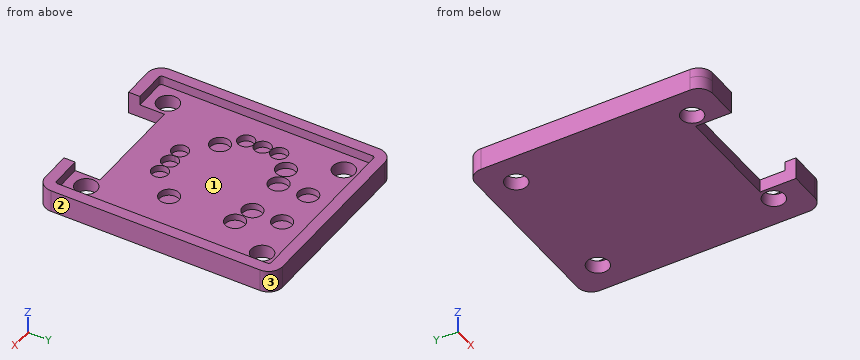
```python
from build123d import *

# Parameters (mm, degrees)
SKETCH002_R   = 1.651
PAD_DEPTH     = 2
SKETCH004_R   = 1.5
SKETCH004_R_2 = 1.25
POCKET_DEPTH  = 1
PAD001_DEPTH  = 1.4


with BuildPart() as part:
    # Sketch002 → Pad (new body)
    with BuildSketch(Plane.XY):
        with BuildLine():
            Line((-2.1, 31.749999), (-2.1, -1e-06))
            ThreePointArc((-2.1, -1e-06), (-1.484924, -1.484925), (0, -2.1))
            Line((4.726249, -2.1), (0, -2.1))
            Line((4.726249, 3.34784), (4.726249, -2.1))
            Line((20.762018, 3.34784), (4.726249, 3.34784))
            Line((20.762018, -2.1), (20.762018, 3.34784))
            Line((20.762018, -2.1), (25.4, -2.1))
            ThreePointArc((25.4, -2.1), (26.884924, -1.484924), (27.5, -1e-06))
            Line((27.5, -1e-06), (27.5, 31.75))
            ThreePointArc((27.5, 31.75), (26.884924, 33.234924), (25.400001, 33.85))
            Line((25.400001, 33.85), (1e-06, 33.85))
            ThreePointArc((1e-06, 33.85), (-1.484924, 33.234924), (-2.1, 31.749999))
        make_face()
        with Locations((2.54, 29.21)):
            Circle(SKETCH002_R, mode=Mode.SUBTRACT)
        with Locations((22.86, 29.21)):
            Circle(SKETCH002_R, mode=Mode.SUBTRACT)
        with Locations((22.86, 2.54)):
            Circle(SKETCH002_R, mode=Mode.SUBTRACT)
        with Locations((2.54, 2.54)):
            Circle(SKETCH002_R, mode=Mode.SUBTRACT)
    extrude(amount=PAD_DEPTH)

    # Sketch004 (on Face18 of Pad) → Pocket (cut)
    with BuildSketch(Plane.XY.offset(2)):
        with Locations((9.45, 28.03)):
            Circle(SKETCH004_R)
        with Locations((15.95, 28.03)):
            Circle(SKETCH004_R)
        with Locations((19.025, 22.78)):
            Circle(SKETCH004_R)
        with Locations((15.95, 23.53)):
            Circle(SKETCH004_R)
        with Locations((9.45, 23.53)):
            Circle(SKETCH004_R)
        with Locations((6.375, 22.78)):
            Circle(SKETCH004_R)
        with Locations((3.97, 20.28)):
            Circle(SKETCH004_R_2)
        with Locations((3.97, 17.78)):
            Circle(SKETCH004_R_2)
        with Locations((3.97, 15.28)):
            Circle(SKETCH004_R_2)
        with Locations((6.375, 12.78)):
            Circle(SKETCH004_R)
        with Locations((10.2, 9.05)):
            Circle(SKETCH004_R_2)
        with Locations((12.7, 9.05)):
            Circle(SKETCH004_R_2)
        with Locations((15.2, 9.05)):
            Circle(SKETCH004_R_2)
        with Locations((19.025, 12.78)):
            Circle(SKETCH004_R)
    extrude(amount=-POCKET_DEPTH, mode=Mode.SUBTRACT)

    # Sketch005 (on Face9 of Pocket) → Pad001 (join)
    with BuildSketch(Plane.XY.offset(2)):
        with BuildLine():
            Line((-2.1, 31.749999), (-2.1, -1e-06))
            ThreePointArc((-2.1, -1e-06), (-1.484924, -1.484924), (0, -2.1))
            Line((4.726249, -2.1), (0, -2.1))
            Line((4.726249, -0.384166), (4.726249, -2.1))
            Line((4.726249, -0.384166), (0, -0.384166))
            ThreePointArc((-0.4, 0.015834), (-0.282843, -0.267009), (0, -0.384166))
            Line((-0.4, 31.75), (-0.4, 0.015834))
            ThreePointArc((0, 32.15), (-0.282843, 32.032843), (-0.4, 31.75))
            Line((25.4, 32.15), (0, 32.15))
            ThreePointArc((25.8, 31.75), (25.682843, 32.032843), (25.4, 32.15))
            Line((25.8, 0), (25.8, 31.75))
            ThreePointArc((25.4, -0.4), (25.682843, -0.282843), (25.8, 0))
            Line((20.762018, -0.4), (25.4, -0.4))
            Line((20.762018, -0.4), (20.762018, -2.1))
            Line((20.762018, -2.1), (25.4, -2.1))
            ThreePointArc((25.4, -2.1), (26.884924, -1.484924), (27.5, -1e-06))
            Line((27.5, -1e-06), (27.5, 31.75))
            ThreePointArc((27.5, 31.75), (26.884924, 33.234924), (25.400001, 33.85))
            Line((25.400001, 33.85), (1e-06, 33.85))
            ThreePointArc((1e-06, 33.85), (-1.484924, 33.234924), (-2.1, 31.749999))
        make_face()
    extrude(amount=PAD001_DEPTH)


solid = part.part
```
Geometry: final body of the model. Coordinates: model frame, mm. Face numbers are marked on the shaded views. Round coordinates to 2 decimals unless told otherwise and drop trailing zeros. Write each loop counter-clockwise with the first axis right and the second up, starting at its lowest first coordinate (ties: lowest second). Pieces come first, ordered by that corner, then holes.
Item 1: Section query D-D (z = 2.55). Return loops of the section in (x, y).
Item 2: Material intervals for L1, parallel to Y at x = 2.54, z = 0.5; L2, parallel to X at y = 20.28, z = 1.45; L3, parallel to Y at x = 21.5, z = 1.15, sorted ascending.
Item 3: Section query A-A (x = 22.86). Return loops of the section in (y, z).
Item 4: Section query C-C (z = 0.6). Return loops of the section in (x, y), plus the area to 3 significant figures.
Item 5: Pin query (flat end, axial travel): P1, Ø12, axis at x = 16, y = 20, coming from the +Z side; P2, Ø1, axis at x = 9.5, z = 1, coming from the -Y side; P3, Ø2.5, axis at x = 6.375, y = 12.78, coming from the +Z side. Return the tip coordinate at first contact, or that it passes through.
Item 6: Mould query, pull axis Y, two halves, no side actions, for the marked faces 1, 2 and 3. Classes: +Y half, -Y half, draft (parallel to the pull), parting line (faces both ways), or undercut.
Item 7: Section query B-B (y = 28.03). Return loops of the section in (x, z), plus the area to 3 significant figures.
Completed:
1. outline: (-2.1, 0) arc R2.1 ccw to (0, -2.1) - (4.73, -2.1) - (4.73, -0.38) - (0, -0.38) arc R0.4 cw to (-0.4, 0.02) - (-0.4, 31.75) arc R0.4 cw to (0, 32.15) - (25.4, 32.15) arc R0.4 cw to (25.8, 31.75) - (25.8, 0) arc R0.4 cw to (25.4, -0.4) - (20.76, -0.4) - (20.76, -2.1) - (25.4, -2.1) arc R2.1 ccw to (27.5, 0) - (27.5, 31.75) arc R2.1 ccw to (25.4, 33.85) - (0, 33.85) arc R2.1 ccw to (-2.1, 31.75) - close
2. L1: y = -2.1 to 0.89, 4.19 to 27.56, 30.86 to 33.85
2. L2: x = -2.1 to 2.72, 5.22 to 27.5
2. L3: y = -2.1 to 1.6, 3.48 to 28.27, 30.15 to 33.85
3. outline: (-2.1, 0) - (0.89, 0) - (0.89, 2) - (-0.4, 2) - (-0.4, 3.4) - (-2.1, 3.4) - close; (4.19, 0) - (27.56, 0) - (27.56, 2) - (4.19, 2) - close; (30.86, 0) - (33.85, 0) - (33.85, 3.4) - (32.15, 3.4) - (32.15, 2) - (30.86, 2) - close
4. outline: (-2.1, 0) arc R2.1 ccw to (0, -2.1) - (4.73, -2.1) - (4.73, 3.35) - (20.76, 3.35) - (20.76, -2.1) - (25.4, -2.1) arc R2.1 ccw to (27.5, 0) - (27.5, 31.75) arc R2.1 ccw to (25.4, 33.85) - (0, 33.85) arc R2.1 ccw to (-2.1, 31.75) - close; hole circle Ø3.3 at (2.54, 2.54); hole circle Ø3.3 at (2.54, 29.21); hole circle Ø3.3 at (22.86, 2.54); hole circle Ø3.3 at (22.86, 29.21)
4. area: 939 mm2
5. P1: stops at z = 2
5. P2: stops at y = 3.35
5. P3: stops at z = 1
6. face 1: undercut
6. face 2: draft
6. face 3: +Y half
7. outline: (-2.1, 0) - (1.39, 0) - (1.39, 2) - (-0.4, 2) - (-0.4, 3.4) - (-2.1, 3.4) - close; (3.69, 0) - (21.71, 0) - (21.71, 2) - (17.45, 2) - (17.45, 1) - (14.45, 1) - (14.45, 2) - (10.95, 2) - (10.95, 1) - (7.95, 1) - (7.95, 2) - (3.69, 2) - close; (24.01, 0) - (27.5, 0) - (27.5, 3.4) - (25.8, 3.4) - (25.8, 2) - (24.01, 2) - close
7. area: 48.7 mm2
